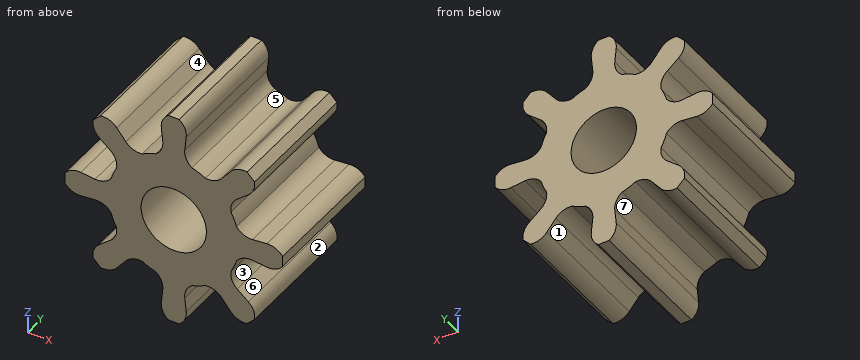
from build123d import *

# Parameters (mm, degrees)
F1_DEPTH = 30
F2_R     = 7.5
F3_DEPTH = 30.001


with BuildPart() as f1:
    # F0 (on Front) → F1 (new body)
    with BuildSketch(Plane.XZ):
        with BuildLine():
            ThreePointArc((-14.555619, 10.982389), (-13.34453, 9.30297), (-13.135405, 7.243005))
            ThreePointArc((-13.135405, 7.243005), (-13.858193, 5.740251), (-14.409712, 4.166556))
            ThreePointArc((-14.409712, 4.166556), (-16.0142, 2.857814), (-18.058099, 2.526655))
            Line((-18.058099, 2.526655), (-21.351614, 2.861007))
            ThreePointArc((-21.351614, 2.861007), (-23.395512, 2.529847), (-25, 1.221105))
            Line((-25, 1.221105), (-25, -1.221105))
            ThreePointArc((-25, -1.221105), (-23.395512, -2.529847), (-21.351614, -2.861007))
            Line((-21.351614, -2.861007), (-18.058099, -2.526655))
            ThreePointArc((-18.058099, -2.526655), (-16.0142, -2.857814), (-14.409712, -4.166556))
            ThreePointArc((-14.409712, -4.166556), (-13.858193, -5.740251), (-13.135405, -7.243005))
            ThreePointArc((-13.135405, -7.243005), (-13.34453, -9.30297), (-14.555619, -10.982389))
            Line((-14.555619, -10.982389), (-17.120908, -13.074834))
            ThreePointArc((-17.120908, -13.074834), (-18.331997, -14.754253), (-18.541121, -16.814218))
            Line((-18.541121, -16.814218), (-16.814218, -18.541121))
            ThreePointArc((-16.814218, -18.541121), (-14.754253, -18.331997), (-13.074834, -17.120908))
            Line((-13.074834, -17.120908), (-10.982389, -14.555619))
            ThreePointArc((-10.982389, -14.555619), (-9.30297, -13.34453), (-7.243005, -13.135405))
            ThreePointArc((-7.243005, -13.135405), (-5.740251, -13.858193), (-4.166556, -14.409712))
            ThreePointArc((-4.166556, -14.409712), (-2.857814, -16.0142), (-2.526655, -18.058099))
            Line((-2.526655, -18.058099), (-2.861007, -21.351614))
            ThreePointArc((-2.861007, -21.351614), (-2.529847, -23.395512), (-1.221105, -25))
            Line((-1.221105, -25), (1.221105, -25))
            ThreePointArc((1.221105, -25), (2.529847, -23.395512), (2.861007, -21.351614))
            Line((2.861007, -21.351614), (2.526655, -18.058099))
            ThreePointArc((2.526655, -18.058099), (2.857814, -16.0142), (4.166556, -14.409712))
            ThreePointArc((4.166556, -14.409712), (5.740251, -13.858193), (7.243005, -13.135405))
            ThreePointArc((7.243005, -13.135405), (9.30297, -13.34453), (10.982389, -14.555619))
            Line((10.982389, -14.555619), (13.074834, -17.120908))
            ThreePointArc((13.074834, -17.120908), (14.754253, -18.331997), (16.814218, -18.541121))
            Line((16.814218, -18.541121), (18.541121, -16.814218))
            ThreePointArc((18.541121, -16.814218), (18.331997, -14.754253), (17.120908, -13.074834))
            Line((17.120908, -13.074834), (14.555619, -10.982389))
            ThreePointArc((14.555619, -10.982389), (13.34453, -9.30297), (13.135405, -7.243005))
            ThreePointArc((13.135405, -7.243005), (13.858193, -5.740251), (14.409712, -4.166556))
            ThreePointArc((14.409712, -4.166556), (16.0142, -2.857814), (18.058099, -2.526655))
            Line((18.058099, -2.526655), (21.351614, -2.861007))
            ThreePointArc((21.351614, -2.861007), (23.395512, -2.529847), (25, -1.221105))
            Line((25, -1.221105), (25, 1.221105))
            ThreePointArc((25, 1.221105), (23.395512, 2.529847), (21.351614, 2.861007))
            Line((21.351614, 2.861007), (18.058099, 2.526655))
            ThreePointArc((18.058099, 2.526655), (16.0142, 2.857814), (14.409712, 4.166556))
            ThreePointArc((14.409712, 4.166556), (13.858193, 5.740251), (13.135405, 7.243005))
            ThreePointArc((13.135405, 7.243005), (13.34453, 9.30297), (14.555619, 10.982389))
            Line((14.555619, 10.982389), (17.120908, 13.074834))
            ThreePointArc((17.120908, 13.074834), (18.331997, 14.754253), (18.541121, 16.814218))
            Line((18.541121, 16.814218), (16.814218, 18.541121))
            ThreePointArc((16.814218, 18.541121), (14.754253, 18.331997), (13.074834, 17.120908))
            Line((13.074834, 17.120908), (10.982389, 14.555619))
            ThreePointArc((10.982389, 14.555619), (9.30297, 13.34453), (7.243005, 13.135405))
            ThreePointArc((7.243005, 13.135405), (5.740251, 13.858193), (4.166556, 14.409712))
            ThreePointArc((4.166556, 14.409712), (2.857814, 16.0142), (2.526655, 18.058099))
            Line((2.526655, 18.058099), (2.861007, 21.351614))
            ThreePointArc((2.861007, 21.351614), (2.529847, 23.395512), (1.221105, 25))
            Line((1.221105, 25), (-1.221105, 25))
            ThreePointArc((-1.221105, 25), (-2.529847, 23.395512), (-2.861007, 21.351614))
            Line((-2.861007, 21.351614), (-2.526655, 18.058099))
            ThreePointArc((-2.526655, 18.058099), (-2.857814, 16.0142), (-4.166556, 14.409712))
            ThreePointArc((-4.166556, 14.409712), (-5.740251, 13.858193), (-7.243005, 13.135405))
            ThreePointArc((-7.243005, 13.135405), (-9.30297, 13.34453), (-10.982389, 14.555619))
            Line((-10.982389, 14.555619), (-13.074834, 17.120908))
            ThreePointArc((-13.074834, 17.120908), (-14.754253, 18.331997), (-16.814218, 18.541121))
            Line((-16.814218, 18.541121), (-18.541121, 16.814218))
            ThreePointArc((-18.541121, 16.814218), (-18.331997, 14.754253), (-17.120908, 13.074834))
            Line((-17.120908, 13.074834), (-14.555619, 10.982389))
        make_face()
    extrude(amount=F1_DEPTH)

    # F2 (on face) → F3 (cut, through all)
    with BuildSketch(Plane.XZ.offset(30)):
        Circle(F2_R)
    extrude(amount=-F3_DEPTH, mode=Mode.SUBTRACT)


solid = f1.part
CAD build for the part. Positions are in the model's coordinates, mm. Face numbers are marked on the shaded views. A direction names the side the tool comes from. Give positions to 0.01 mm unless a question says otherwise; leave off trailing zeros. Order: outer loops, then holes, each group sorted by start corner. A loop starts at its lowest first (then second) coordinate and runs counter-clockwise, first axis right, second up. Notation, with made-up numbers: (5, -30) - (21, -30) arc R16 ccw to (21, -9) - close; hole circle Ø9 at (49, 27.25). An arc over 180 degrees is marked (long way). Answer in a Markdown table with one row per item.
1. Tool access for the marked faces 5, 6 and 7: list every direction of +Z, -Z, +X, -X, +Y, -Y with a clear straight run to the whole face (end or side of a thin tool).
Data:
| item | result |
|---|---|
| face 5 | +Z, +Y, -Y |
| face 6 | +X, +Y, -Y |
| face 7 | +Y, -Y |
2. Saw through at D-D, the plane x = -10. Give the cut face in (y, z).
Data:
| item | result |
|---|---|
| outline | (-30, -13.69) - (0, -13.69) - (0, 13.69) - (-30, 13.69) - close |
3. Saw through at C-C, the plane z = 12. Give the cut face in (x, y), plus the area to 3 significant figures.
Data:
| item | result |
|---|---|
| outline | (-15.8, -30) - (15.8, -30) - (15.8, 0) - (-15.8, 0) - close |
| area | 948 mm² |
4. Flat gauge pins, fed straight in: pin 1 (6 mm diameter, centred on y = -16.5, z = 18, fed in from +X); pin 2 (9 mm diameter, centred on x = 0, z = 0, fed in from +Y); pin 3 (5 mm diameter, centred on x = 17, y = -11.5, fed in from -Z); pin 4 (1.5 mm diameter, centred on y = -15.5, z = 5, fed in from +X). Where does each tip first touch, or does it go through?
Data:
| item | result |
|---|---|
| pin 1 | stops at x = 18.59 |
| pin 2 | passes through |
| pin 3 | stops at z = -18.59 |
| pin 4 | stops at x = 14.39 |
5. Saw through at B-B, the plane z = 0. Give the cut face in (x, y).
Data:
| item | result |
|---|---|
| outline | (-25, -30) - (-7.5, -30) - (-7.5, 0) - (-25, 0) - close; (7.5, -30) - (25, -30) - (25, 0) - (7.5, 0) - close |
6. Pull direction Z, two halves, no side cores. Call the marked faces 1, 2, 3 and 4: pulls with the +Z half, pulls with the -Z half, needs draft (parallel to the pull), parting line crosses it, or undercut.
Data:
| item | result |
|---|---|
| face 1 | pulls with the -Z half |
| face 2 | undercut |
| face 3 | undercut |
| face 4 | pulls with the +Z half |
7. Saw through at A-A, the plane x = 0. Give the cut face in (y, z), plus the area to 3 significant figures.
Data:
| item | result |
|---|---|
| outline | (-30, -25) - (0, -25) - (0, -7.5) - (-30, -7.5) - close; (-30, 7.5) - (0, 7.5) - (0, 25) - (-30, 25) - close |
| area | 1,050 mm² |
8. Probe probe 1 along Z at (x, y) = (0, -21.5); probe 2 along X at (y, z) = (-14, -15.5); probe 3 along Z at (x, y) = (14.5, -2.5). List the from-to ranges inside material, lowest first. Write a range as [from, to].
Data:
| item | result |
|---|---|
| probe 1 | z = [-25, -7.5], [7.5, 25] |
| probe 2 | x = [-18.54, -11.75], [-3.14, 3.14], [11.75, 18.54] |
| probe 3 | z = [-18.23, -10.94], [-4.05, 4.05], [10.94, 18.23] |
